from build123d import *

# Parameters (mm, degrees)
SKETCH_1_R      = 1.1
EXTRUDE_1_DEPTH = 1.6
SKETCH_2_W      = 4.6
SKETCH_2_H      = 8.8
EXTRUDE_2_DEPTH = 6
SKETCH_3_W      = 5.2
SKETCH_3_H      = 10
EXTRUDE_3_DEPTH = 8


with BuildPart() as part:
    # ｽｹｯﾁ1 → ﾎﾞｽ - 押し出し1 (new body)
    with BuildSketch(Plane(origin=(0, 0, 0), x_dir=(0, 1, 0), z_dir=(0, 0, 1))):
        with BuildLine():
            Line((0, 8), (0, 0))
            Line((0, 0), (20, 0))
            Line((20, 0), (20, 8))
            ThreePointArc((20, 8), (22, 10), (20, 12))
            Line((20, 12), (20, 20))
            Line((20, 20), (12.5, 20))
            ThreePointArc((12.5, 20), (10, 17.5), (7.5, 20))
            Line((7.5, 20), (0, 20))
            Line((0, 20), (0, 12))
            ThreePointArc((0, 12), (-2, 10), (0, 8))
        make_face()
        with Locations((20, 10)):
            Circle(SKETCH_1_R, mode=Mode.SUBTRACT)
        with Locations((0, 10)):
            Circle(SKETCH_1_R, mode=Mode.SUBTRACT)
    extrude(amount=EXTRUDE_1_DEPTH)

    # ｽｹｯﾁ2 → ﾎﾞｽ - 押し出し2 (add)
    with BuildSketch(Plane(origin=(0, 0, 0), x_dir=(1, 0, 0), z_dir=(0, 0, -1))):
        with Locations((-15.1, -10)):
            Rectangle(SKETCH_2_W, SKETCH_2_H)
    extrude(amount=EXTRUDE_2_DEPTH)

    # ｽｹｯﾁ3 → ﾎﾞｽ - 押し出し3 (add)
    with BuildSketch(Plane.XY.offset(1.6)):
        with Locations((-3.6, 10)):
            Rectangle(SKETCH_3_W, SKETCH_3_H)
    extrude(amount=EXTRUDE_3_DEPTH)


solid = part.part
Can you work these out from the model? Positions are in its coordinate system, mm. A direction names the side the tool comes from. Give positions to 0.01 mm unless a question says otherwise; leave off trailing zeros. Loops run counter-clockwise (first coordinate to the right, second up) from the corner with the lowest first, then second, coordinate; pieces in that order, holes last. Notation, with made-up numbers: (13, 2) - (56, 2) arc R4 cw to (56, 8) - close; hole circle Ø1 at (-35, -39.5). An arc over 180 degrees is marked (long way). Answer as a JSON object with one key per item and string values.
Q1. Imagine slicing it at D-D on y = 13.5. Write out the boundary of the cut face in (x, z).
Geometry says:
{"outline": "(-20, 0) - (-17.4, 0) - (-17.4, -6) - (-12.8, -6) - (-12.8, 0) - (0, 0) - (0, 1.6) - (-1, 1.6) - (-1, 9.6) - (-6.2, 9.6) - (-6.2, 1.6) - (-20, 1.6) - close"}
Q2. If we mould it in two halves opening along X, with no side actions, what happens to faces 4 (the flat face through (-16, 20, 1)), 5 (the cylindrical face through (-8.926, -0.238, 0.789)), 6 (the cylindrical face through (-10, -2, 1))? For each: pulls with the +X half, pulls with the -X half, needs draft (parallel to the pull), parting line crosses it, or undercut.
Geometry says:
{"face 4": "needs draft", "face 5": "undercut", "face 6": "parting line crosses it"}
Q3. Which directions (+Z, -Z, +X, -X, +Y, -Y) give clear straight access to the entire face, cutting with the end or side of a thin tool? Please do faces 1 (the flat face through (-4, 0, 1)), 2 (the flat face through (-16, 0, 1)), 3 (the flat face through (-4, 15, 6)).
Geometry says:
{"face 1": "+Z, -Z, +X, -Y", "face 2": "+Z, -Z, -X, -Y", "face 3": "+Z, +X, -X, +Y"}
Q4. Imagine slicing it at C-C on z = -1.25. Write out the boundary of the cut face in (x, y), plus the area to 3 significant figures.
Geometry says:
{"outline": "(-17.4, 5.6) - (-12.8, 5.6) - (-12.8, 14.4) - (-17.4, 14.4) - close", "area": "40.5 mm²"}
Q5. Will these pins go through, and if not, where does the flat tip stop? P1, Ø2, axis at x = -13.5, z = -2, coming from the -Y side; P2, Ø1, axis at x = -13, y = 18, coming from the +Z side; P3, Ø3.5, axis at x = -15.5, z = -3, coming from the +Y side; P4, Ø8, axis at y = 18, z = -2.5, coming from the -X side.
Geometry says:
{"P1": "y = 5.6", "P2": "z = 1.6", "P3": "y = 14.4", "P4": "x = -20"}
Q6. Imagine slicing it at B-B on x = -4. Write out the boundary of the cut face in (y, z), plus the area to 3 significant figures.
Geometry says:
{"outline": "(0, 0) - (20, 0) - (20, 1.6) - (15, 1.6) - (15, 9.6) - (5, 9.6) - (5, 1.6) - (0, 1.6) - close", "area": "112 mm²"}
Q7. If I drill on L1, parallel to Y at x = -10, z = 0.95; L2, parallel to Z at x = -5.5, y = 4.5; L3, parallel to X at y = 9, z = -3.25, over which ranges is the centre line in solid material (lowest first)?
Geometry says:
{"L1": "-2 to -1.1, 1.1 to 18.9, 21.1 to 22", "L2": "0 to 1.6", "L3": "-17.4 to -12.8"}
Q8. Imagine slicing it at A-A on y = 8.5. Write out the boundary of the cut face in (x, z), plus the area to 3 significant figures.
Geometry says:
{"outline": "(-18, 0) - (-17.4, 0) - (-17.4, -6) - (-12.8, -6) - (-12.8, 0) - (0, 0) - (0, 1.6) - (-1, 1.6) - (-1, 9.6) - (-6.2, 9.6) - (-6.2, 1.6) - (-18, 1.6) - close", "area": "98.0 mm²"}
